Job drawing, mm, ordinate dimensions from the low corner. One solid piece. Round coordinates to 2 decimals unless told otherwise and drop trailing zeros. Order: outer loops, then holes, each group sorted by start corner. A loop starts at its lowest first (then second) coordinate and runs counter-clockwise, first axis right, second up. Notation, with made-up numbers: (28.5, -17.5) - (69.5, -17.5) arc R24 cw to (69.5, 10.5) - close; hole circle Ø11 at (58.25, 67). An arc over 180 degrees is marked (long way). Use one line per item in the form item = value. Start each with the question number.
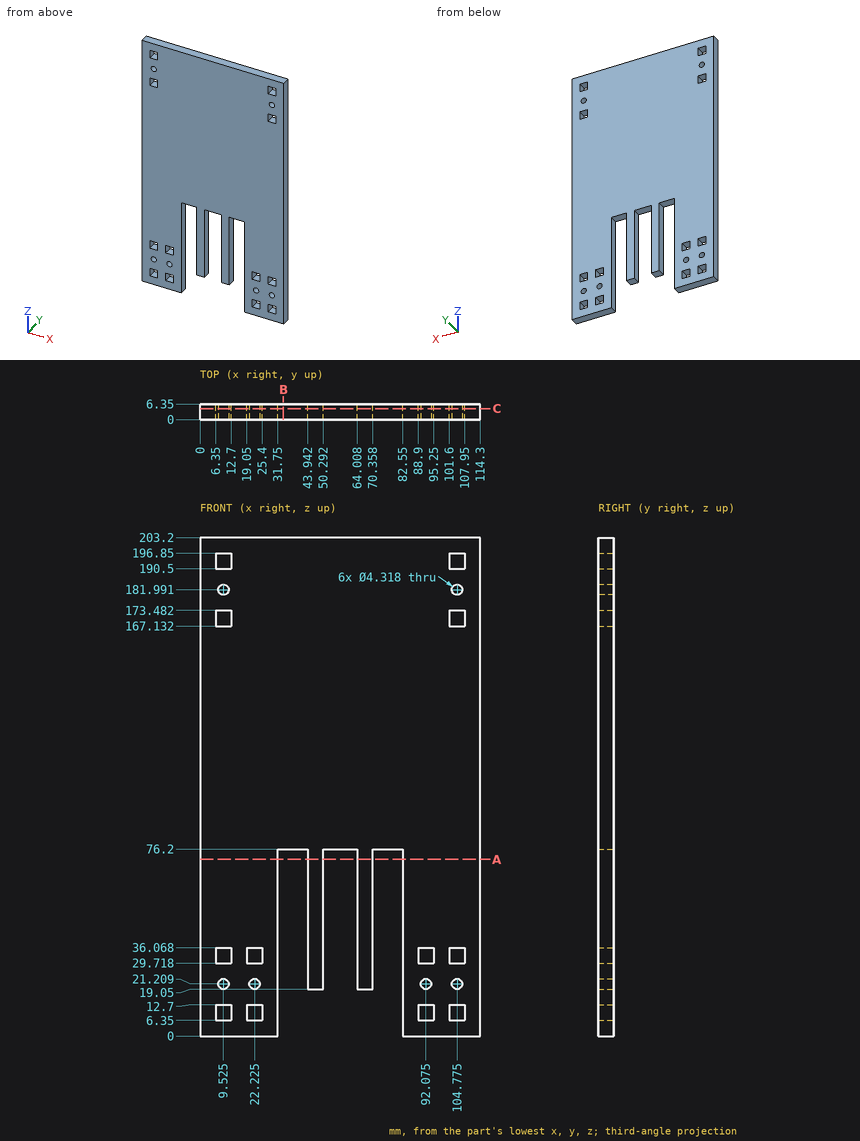
(1) Flat gauge pins, fed straight in: P1, Ø6, axis at x = 79.5, z = 40.5, coming from the +Y side; P2, Ø3, axis at x = 44.5, y = 5.5, coming from the -Z side. Where does each tip first touch, or does it go through?
(2) Slice it at A-A (z = 72). Give the cut face in (x, y).
(3) Slice it at C-C (y = 4.5). Give the number of separate pieces and of enclosed holes in the cut face, and give its area (3 significant figures).
(4) Wall check: line 1 (Z direction, x = 102.5, y = 0.75); line 2 (X direction, y = 1.25, z = 60); line 3 (X direction, y = 1.5, z = 191). Give the ranges that are in metal, low to high. Write a range as [from, to].
(5) Slice it at B-B (x = 34). Give the cut face in (y, z).
Results list:
q1.P1 = through
q1.P2 = 19.05
q2.outline = (0, 0) - (31.75, 0) - (31.75, 6.35) - (0, 6.35) - close; (43.94, 0) - (50.29, 0) - (50.29, 6.35) - (43.94, 6.35) - close; (64.01, 0) - (70.36, 0) - (70.36, 6.35) - (64.01, 6.35) - close; (82.55, 0) - (114.3, 0) - (114.3, 6.35) - (82.55, 6.35) - close
q3.separate_pieces = 1
q3.enclosed_holes = 18
q3.area = 19,500 mm²
q4.line_1 = [0, 6.35], [12.7, 29.72], [36.07, 167.13], [173.48, 190.5], [196.85, 203.2]
q4.line_2 = [0, 31.75], [43.94, 50.29], [64.01, 70.36], [82.55, 114.3]
q4.line_3 = [0, 6.35], [12.7, 101.6], [107.95, 114.3]
q5.outline = (0, 76.2) - (6.35, 76.2) - (6.35, 203.2) - (0, 203.2) - close
